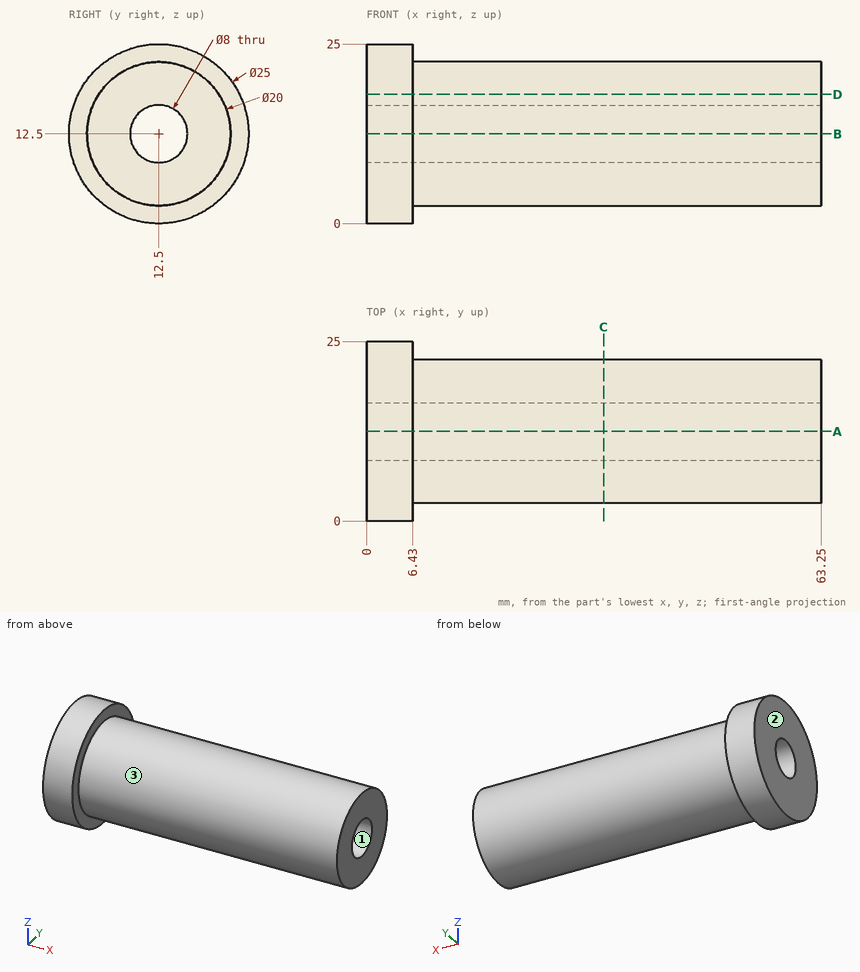
Source: three-view drawing plus pictorial views. Frame: mm from the lowest corner of the part. Coordinates: 2 decimals unless noted, no trailing zeros. Order: outer loops, then holes, each group sorted by start corner. A loop starts at its lowest first (then second) coordinate and runs counter-clockwise, first axis right, second up. Notation, with made-up numbers: M 68.25,18.5 L 93.25,18.5 A34 cw 93.25,53.5 Z; hole C 83.25,20 d11. An arc over 180 degrees is marked long. Write each question's results on one line, items separated by ' | '. Start each with the question number.
1. Section A-A, the plane y = 12.5. Return the cut outline in (x, z).
2. Section C-C, the plane x = 33. Return the cut outline in (y, z).
3. Draft query along Y for the marked faces 1, 2 and 3. Return one class per face: +Y half, -Y half, draft (parallel to the pull), parting line (faces both ways), or undercut.
4. Section D-D, the plane z = 18. Return the cut outline in (x, y), then the cut area to 3 significant figures.
5. Pin query (flat end, axial travel): pin 1 (12 mm diameter, centred on x = 29.5, z = 4, fed in from -Y); pin 2 (10 mm diameter, centred on y = 11, z = 2.5, fed in from -X); pin 3 (2 mm diameter, centred on x = 47.5, y = 7.5, fed in from -Z); pin 4 (3 mm diameter, centred on x = 26, y = 5, fed in from -Z). Return the tip coordinate at first contact, or that it passes through.
6. Material intervals for L1, parallel to Y at x = 41.5, z = 12.5; L2, parallel to X at y = 2, z = 16.5; L3, parallel to Y at x = 54, z = 14.25, sorted ascending.
Solution:
1) outline: M 0,0 L 6.43,0 L 6.43,2.5 L 63.25,2.5 L 63.25,8.5 L 0,8.5 Z; M 0,16.5 L 63.25,16.5 L 63.25,22.5 L 6.43,22.5 L 6.43,25 L 0,25 Z
2) outline: C 12.5,12.5 d20; hole C 12.5,12.5 d8
3) face 1: undercut | face 2: draft | face 3: parting line
4) outline: M 0,1.28 L 6.43,1.28 L 6.43,4.15 L 63.25,4.15 L 63.25,20.85 L 6.43,20.85 L 6.43,23.72 L 0,23.72 Z | area: 1,090 mm²
5) pin 1: y = 2.82 | pin 2: x = 0 | pin 3: z = 3.33 | pin 4: z = 4.5
6) L1: 2.5 to 8.5, 16.5 to 22.5 | L2: 0 to 6.43 | L3: 2.65 to 8.9, 16.1 to 22.35
